Can you work these out from the model? Positions are in its coordinate system, mm. Round coordinates to 2 decimals unless told otherwise and drop trailing zeros. Loops run counter-clockwise (first coordinate to the right, second up) from the corner with the lowest first, then second, coordinate; pieces in that order, holes last.
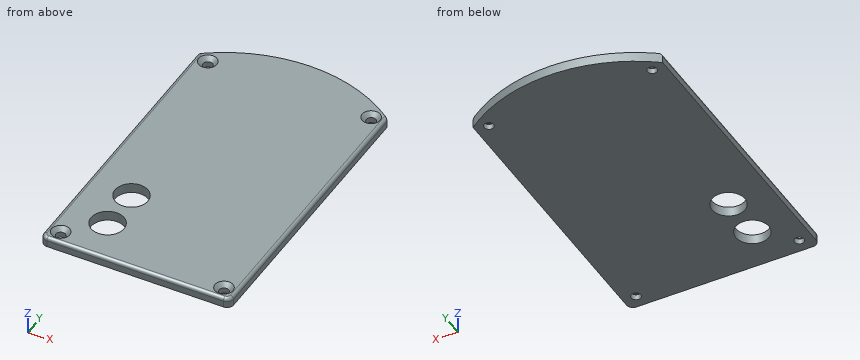
from build123d import *

# Parameters (mm, degrees)
SCHIZZO4_W                               = 57.5
SCHIZZO4_H                               = 100
ESTRUSIONE_ESTRUSIONE2_DEPTH             = 3
TAGLIO_ESTRUSIONE2_REACH                 = 59.754
SCHIZZO7_R                               = 5
RACCORDO1_R                              = 2
RACCORDO3_R                              = 2
RACCORDO4_R                              = 1
FORO_SVASATO_PER_VITE_M2_5_1_D           = 2.9
FORO_SVASATO_PER_VITE_M2_5_1_CSINK_D     = 5.5
FORO_SVASATO_PER_VITE_M2_5_1_CSINK_ANGLE = 90


with BuildPart() as part:
    # Schizzo4 → Estrusione-Estrusione2 (new body)
    with BuildSketch(Plane.XY):
        Rectangle(SCHIZZO4_W, SCHIZZO4_H)
    extrude(amount=ESTRUSIONE_ESTRUSIONE2_DEPTH)

    # Schizzo7 → Taglio-Estrusione2 (cut, up to next)
    with BuildSketch(Plane.XY, mode=Mode.PRIVATE) as taglio_estrusione2_sk1:
        with Locations(Location((-15.52, -36.81, 0), (0, 0, 180))):
            Circle(SCHIZZO7_R)
    taglio_estrusione2_tool1 = extrude(taglio_estrusione2_sk1.sketch, amount=TAGLIO_ESTRUSIONE2_REACH, mode=Mode.PRIVATE) & part.part
    # Schizzo7 → Taglio-Estrusione2 (cut, up to next)
    with BuildSketch(Plane.XY, mode=Mode.PRIVATE) as taglio_estrusione2_sk2:
        with Locations(Location((-15.52, -23.47, 0), (0, 0, 180))):
            Circle(SCHIZZO7_R)
    taglio_estrusione2_tool2 = extrude(taglio_estrusione2_sk2.sketch, amount=TAGLIO_ESTRUSIONE2_REACH, mode=Mode.PRIVATE) & part.part
    # Schizzo7 → Taglio-Estrusione2 (cut, up to next)
    with BuildSketch(Plane.XY, mode=Mode.PRIVATE) as taglio_estrusione2_sk3:
        with BuildLine():
            Line((-28.75, 37.61), (-28.75, 50))
            Line((-28.75, 50), (28.75, 50))
            Line((28.75, 50), (28.75, 37.61))
            ThreePointArc((28.75, 37.61), (0, 47.339989438), (-28.75, 37.61))
        make_face()
    taglio_estrusione2_tool3 = extrude(taglio_estrusione2_sk3.sketch, amount=TAGLIO_ESTRUSIONE2_REACH, mode=Mode.PRIVATE) & part.part
    add(taglio_estrusione2_tool1.solids().sort_by_distance((-15.52, -36.81, 0))[0], mode=Mode.SUBTRACT)
    add(taglio_estrusione2_tool2.solids().sort_by_distance((-15.52, -23.47, 0))[0], mode=Mode.SUBTRACT)
    add(taglio_estrusione2_tool3.solids().sort_by_distance((-28.161803, 43.805, 0))[0], mode=Mode.SUBTRACT)

    # Raccordo1
    raccordo1_edges = [part.edges().sort_by_distance(p)[0] for p in [
        (-28.75, -50, 1.5),
    ]]
    fillet(raccordo1_edges, radius=RACCORDO1_R)

    # Raccordo3
    raccordo3_edges = [part.edges().sort_by_distance(p)[0] for p in [
        (28.75, -50, 1.5),
    ]]
    fillet(raccordo3_edges, radius=RACCORDO3_R)

    # Raccordo4
    raccordo4_edges = [part.edges().sort_by_distance(p)[0] for p in [
        (-28.75, -5.195, 3),
        (0, -50, 3),
        (-28.164213562, -49.414213562, 3),
        (28.75, -5.195, 3),
        (28.164213562, -49.414213562, 3),
    ]]
    fillet(raccordo4_edges, radius=RACCORDO4_R)

    # Foro svasato per Vite M2.5-1 (through all)
    with Locations(Plane.XY.offset(3)):
        with Locations((-24.75, 36.11), (24.75, -46), (-24.75, -46), (24.75, 36.11)):
            CounterSinkHole(FORO_SVASATO_PER_VITE_M2_5_1_D / 2, FORO_SVASATO_PER_VITE_M2_5_1_CSINK_D / 2, counter_sink_angle=FORO_SVASATO_PER_VITE_M2_5_1_CSINK_ANGLE)


solid = part.part
(1) If we section it at B-B, the plane y = 36.11: List the corners of the cut face in (x, z) for me, then the cut area to 3 significant figures.
Worked answers:
outline: (-28.75, 0) - (-26.2, 0) - (-26.2, 1.7) - (-27.5, 3) - (-27.75, 3) arc R1 ccw to (-28.75, 2) - close; (-23.3, 0) - (23.3, 0) - (23.3, 1.7) - (22, 3) - (-22, 3) - (-23.3, 1.7) - close; (26.2, 0) - (28.75, 0) - (28.75, 2) arc R1 ccw to (27.75, 3) - (27.5, 3) - (26.2, 1.7) - close
area: 151 mm2
(2) Will this pin go through, and if not, where does the flat tip stop? P1, Ø2.5, axis at x = 24.75, y = 36.11, coming from the +Z side (1 decimal).
Worked answers:
P1: passes through
(3) If we section it at C-C, the plane x = -24.75: List the corners of the cut face in (y, z) for me, then the cut area to 3 significant figures.
Worked answers:
outline: (-50, 0) - (-47.45, 0) - (-47.45, 1.7) - (-48.75, 3) - (-49, 3) arc R1 ccw to (-50, 2) - close; (-44.55, 0) - (34.66, 0) - (34.66, 1.7) - (33.36, 3) - (-43.25, 3) - (-44.55, 1.7) - close; (37.56, 0) - (40.35, 0) - (40.35, 3) - (38.86, 3) - (37.56, 1.7) - close
area: 250 mm2
(4) If we section it at A-A, the plane y = -36.81: List the corners of the cut face in (x, z) for me.
Worked answers:
outline: (-28.75, 0) - (-20.52, 0) - (-20.52, 3) - (-27.75, 3) arc R1 ccw to (-28.75, 2) - close; (-10.52, 0) - (28.75, 0) - (28.75, 2) arc R1 ccw to (27.75, 3) - (-10.52, 3) - close
(5) If I drill on line 1 (X direction, y = -36.81, z = 1.05); line 2 (X direction, y = -45, z = 0.25); line 3 (Y direction, x = -24.75, z = 0.8), over which ranges is the centre line in solid material (lowest first)?
Worked answers:
line 1: x = -28.75 to -20.52, -10.52 to 28.75
line 2: x = -28.75 to -25.8, -23.7 to 23.7, 25.8 to 28.75
line 3: y = -50 to -47.45, -44.55 to 34.66, 37.56 to 40.35
(6) If we section it at D-D, the plane x = -15.52: List the corners of the cut face in (y, z) for me, then the cut area to 3 significant figures.
Worked answers:
outline: (-50, 0) - (-41.81, 0) - (-41.81, 3) - (-49, 3) arc R1 ccw to (-50, 2) - close; (-31.81, 0) - (-28.47, 0) - (-28.47, 3) - (-31.81, 3) - close; (-18.47, 0) - (44.72, 0) - (44.72, 3) - (-18.47, 3) - close
area: 224 mm2
